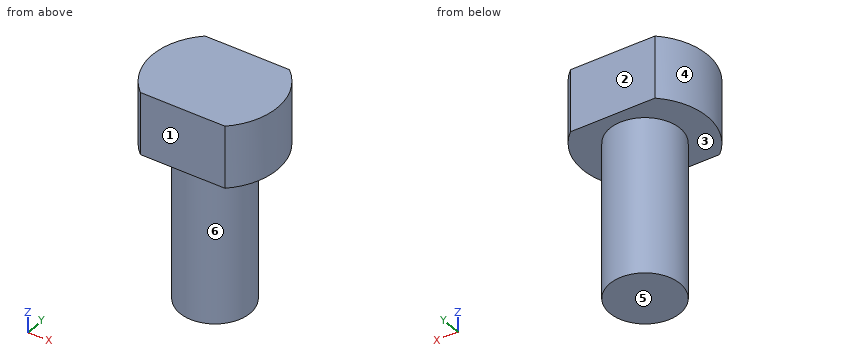
from build123d import *

# Parameters (mm, degrees)
SKETCH1_R           = 2.25
BOSS_EXTRUDE1_DEPTH = 10
SKETCH2_R           = 4
BOSS_EXTRUDE2_DEPTH = 4
CUT_EXTRUDE1_START  = -4
CUT_EXTRUDE1_DEPTH  = 4


with BuildPart() as part:
    # Sketch1 → Boss-Extrude1 (new body)
    with BuildSketch(Plane.XY):
        Circle(SKETCH1_R)
    extrude(amount=BOSS_EXTRUDE1_DEPTH)

    # Sketch2 → Boss-Extrude2 (add)
    with BuildSketch(Plane.XY.offset(10)):
        Circle(SKETCH2_R)
    extrude(amount=BOSS_EXTRUDE2_DEPTH)

    # Sketch3 → Cut-Extrude1 (cut)
    with BuildSketch(Plane.XY.offset(14).offset(CUT_EXTRUDE1_START)):
        with BuildLine():
            Line((-2.645751311, 3), (2.645751311, 3))
            ThreePointArc((2.645751311, 3), (0, 4), (-2.645751311, 3))
        make_face()
        with BuildLine():
            Line((-2.645751311, -3), (2.645751311, -3))
            ThreePointArc((2.645751311, -3), (0, -4), (-2.645751311, -3))
        make_face()
    extrude(amount=CUT_EXTRUDE1_DEPTH, mode=Mode.SUBTRACT)


solid = part.part
Read the model definition and answer for the solid it produces. Units are mm, in the model's axes. Face numbers are marked on the shaded views. A direction names the side the tool comes from. Give positions to 0.01 mm unless a question says otherwise; leave off trailing zeros. Loops run counter-clockwise (first coordinate to the right, second up) from the corner with the lowest first, then second, coordinate; pieces in that order, holes last. Notation, with made-up numbers: (-9, -18.5) -> (15, -18.5) arc R5 cw to (15, -14.5) -> close; hole circle Ø10 at (-27, 20). An arc over 180 degrees is marked (long way). Answer as CSV lines item,"result".
Item 1: Determine the mould class of the marked faces 1, 2, 3 and 4 for opening direction Y: +Y half, -Y half, draft (parallel to the pull), parting line (faces both ways), or undercut.
Returned:
face 1,"-Y half"
face 2,"+Y half"
face 3,"draft"
face 4,"parting line"
Item 2: Each of these flat-tipped pins is pushed along its axis until it touches: pin 1 (4 mm diameter, centred on x = -2, z = 4, fed in from -Y); pin 2 (3 mm diameter, centred on y = -1, z = 3.5, fed in from +X). Where does it stop, or does it pass through?
Returned:
pin 1,"stops at y = -2.25"
pin 2,"stops at x = 2.25"
Item 3: Find section A-A on y = 0. Give the vertices of the cut face in (x, z).
Returned:
outline,"(-4, 10) -> (-2.25, 10) -> (-2.25, 0) -> (2.25, 0) -> (2.25, 10) -> (4, 10) -> (4, 14) -> (-4, 14) -> close"
Item 4: Consider line 1 (Z direction, x = 1.5, y = 1.75); line 2 (X direction, y = 1.25, z = 5.75); line 3 (Y direction, x = 2.75, z = 10.25). Determine where each line is inside the solid, lowest interval first. Write a range as [from, to].
Returned:
line 1,"z = [10, 14]"
line 2,"x = [-1.87, 1.87]"
line 3,"y = [-2.9, 2.9]"
Item 5: Find section D-D on z = 10.25. Give the vertices of the cut face in (x, y), plus the area to 3 significant figures.
Returned:
outline,"(-2.65, -3) -> (2.65, -3) arc R4 ccw to (2.65, 3) -> (-2.65, 3) arc R4 ccw to start"
area,"43.0 mm²"
Item 6: Find section B-B on x = 0. Give the vertices of the cut face in (y, z).
Returned:
outline,"(-3, 10) -> (-2.25, 10) -> (-2.25, 0) -> (2.25, 0) -> (2.25, 10) -> (3, 10) -> (3, 14) -> (-3, 14) -> close"
Item 7: Find section C-C on z = 1.25. Give the vertices of the cut face in (x, y).
Returned:
outline,"circle Ø4.5 at (0, 0)"
Item 8: For the marked faces 5 and 6, determine the directions among +Z, -Z, +X, -X, +Y, -Y from which every point of the face is accessible in a straight line to the end or side of a thin tool.
Returned:
face 5,"-Z, +X, -X, +Y, -Y"
face 6,"-Z"
